Autodesk Fusion 360 part; units mm, degrees
sketch "Sketch1" plane through (0, 0, 0) normal (0, 0, 1) x (1, 0, 0)
  line L0 (68.385, 0) -> (68.385, -31.04)
  line L1 (44.135, 0) -> (44.135, -31.04)
  line L2 (68.385, -31.525) -> (68.385, -31.04)
  line L3 (44.135, -31.525) -> (44.135, -31.04)
  line L4 (-68.385, 0) -> (-68.385, -31.04)
  line L5 (-44.135, 0) -> (-44.135, -31.04)
  line L6 (-68.385, -31.525) -> (-68.385, -31.04)
  line L7 (-44.135, -31.525) -> (-44.135, -31.04)
  arc A0 (44.135, 0) -> (-44.135, 0) centre (0, 0) ccw
  arc A1 (68.385, 0) -> (-68.385, 0) centre (0, 0) ccw
  arc A2 (44.135, -31.525) -> (68.385, -31.525) centre (56.26, -31.525) ccw
  arc A3 (-68.385, -31.525) -> (-44.135, -31.525) centre (-56.26, -31.525) ccw
extrude "Extrude5" add sketch "Sketch1" along normal blind 6
sketch "Sketch4" plane through (0, 0, 0) normal (0, 0, 1) x (1, 0, 0)
sketch "Sketch5" plane through (0, 0, 6) normal (0, 0, 1) x (-1, 0, 0)
  arc A0 (-68.385, 0) -> (68.385, 0) centre (0, 0) ccw
  line L0 (68.385, 0) -> (68.385, 31.525)
  arc A1 (68.385, 31.525) -> (44.135, 31.525) centre (56.26, 31.525) ccw
  line L1 (44.135, 31.525) -> (44.135, 0)
  arc A2 (-44.135, 0) -> (44.135, 0) centre (0, 0) ccw
  line L2 (-44.135, 0) -> (-44.135, 31.525)
  arc A3 (-44.135, 31.525) -> (-68.385, 31.525) centre (-56.26, 31.525) ccw
  line L3 (-68.385, 31.525) -> (-68.385, 0)
  circle A4 centre (56.26, 31.525) radius 2.75
  circle A5 centre (-56.26, 31.525) radius 2.75
  circle A6 centre (0, -63) radius 2.75
  dimension "d79" = 5.5
  dimension "d80" = 5.5
  dimension "d82" = 5.5
extrude "Extrude6" cut sketch "Sketch5" against normal blind 6 contours A4 | A5 | A6
Part model, mm, in its own coordinate system. A direction names the side the tool comes from. Round coordinates to 2 decimals unless told otherwise and drop trailing zeros. Write each loop counter-clockwise with the first axis right and the second up, starting at its lowest first coordinate (ties: lowest second). Pieces come first, ordered by that corner, then holes. Notation, with made-up numbers: M -37,46 L 9,46 A12 cw 9,64 Z; hole C 12.5,1.5 d6. An arc over 180 degrees is marked long. One line per question, with ' | ' between items.
(1) Saw through at A-A on y = -25.5. Write the cut outline in (x, z) (3 decimals), then the cut area to 3 significant figures.
Answer key:
outline: M -68.385,0 L -44.135,0 L -44.135,6 L -68.385,6 Z; M 44.135,0 L 68.385,0 L 68.385,6 L 44.135,6 Z | area: 291 mm^2
(2) Saw through at B-B on x = 0. Write the cut outline in (y, z) (3 decimals), then the cut area to 4 significant figures.
Answer key:
outline: M 44.135,0 L 60.25,0 L 60.25,6 L 44.135,6 Z; M 65.75,0 L 68.385,0 L 68.385,6 L 65.75,6 Z | area: 112.5 mm^2
(3) Pin check, flat tips, straight feed: pin 1 (4.5 mm diameter, centred on x = -56.26, y = -31.525, fed in from -Z); pin 2 (1 mm diameter, centred on y = 6, z = 5, fed in from -X); pin 3 (1 mm diameter, centred on y = 32.5, z = 4, fed in from -X); pin 4 (7 mm diameter, centred on x = 56.26, y = -31.525, fed in from +Z). Stop position of each tip, or through.
Answer key:
pin 1: passes through | pin 2: stops at x = -68.16 | pin 3: stops at x = -60.44 | pin 4: stops at z = 6
(4) Saw through at D-D on x = -17.5. Write the cut outline in (y, z).
Answer key:
outline: M 40.52,0 L 66.11,0 L 66.11,6 L 40.52,6 Z
(5) Two-plate mould, pull along X, no slides. Class faces 1 (the face through (-0.971, 44.124, 2.958)), 2 (the face through (-1, 50, 0)), 3 (the face through (-1.5, 68.37, 2.96)): released by +X, released by -X, zero draft, split by the parting line, or undercut.
Answer key:
face 1: undercut | face 2: zero draft | face 3: split by the parting line
(6) Probe line 1 along X through (y, z) = (-13.5, 0.35) (3 decimals); line 2 along Y through (x, z) = (0, 2.4) (3 decimals); line 3 along X through (y, z) = (-29, 0.65) (3 decimals). List the from-to ranges inside material, lowest first.
Answer key:
line 1: x = -68.385 to -44.135, 44.135 to 68.385 | line 2: y = 44.135 to 60.25, 65.75 to 68.385 | line 3: x = -68.385 to -57.349, -55.171 to -44.135, 44.135 to 55.171, 57.349 to 68.385
(7) 3-axis set-ups, long thin cutter, end or side, ignore diameter. For faces 4 (the face through (0.358, 60.273, 3.042)), 5 (the face through (44.135, -16, 3)): which of +Z, -Z, +X, -X, +Y, -Y reach the whole face in a straight line?
Answer key:
face 4: +Z, -Z | face 5: +Z, -Z, -Y
(8) Saw through at C-C on z = 4.8. Write the cut outline in (x, y) (3 decimals).
Answer key:
outline: M -68.385,-31.525 A12.125 ccw -44.135,-31.525 L -44.135,0 A44.135 cw 44.135,0 L 44.135,-31.525 A12.125 ccw 68.385,-31.525 L 68.385,0 A68.385 ccw -68.385,0 Z; hole C -56.26,-31.525 d5.5; hole C 0,63 d5.5; hole C 56.26,-31.525 d5.5
